```python
from build123d import *

# Parameters (mm, degrees)
BOSS_EXTRUDE1_DEPTH = 7.5
FILLET1_R           = 2.5
SKETCH3_R           = 16.5
BOSS_EXTRUDE2_DEPTH = 5
BOSS_EXTRUDE3_START = -5
BOSS_EXTRUDE3_DEPTH = 5
SKETCH5_R           = 5
BOSS_EXTRUDE4_DEPTH = 10
SKETCH6_R           = 5
CUT_EXTRUDE1_DEPTH  = 10


with BuildPart() as part:
    # Sketch2 → Boss-Extrude1 (new, symmetric)
    with BuildSketch(Plane.XY):
        with BuildLine():
            ThreePointArc((102.783087905, 14.977902914), (19.214406157, 13.934366249), (-64.149557364, 19.872642429))
            ThreePointArc((-64.149557364, 19.872642429), (-86.204808933, 2.808746854), (-69.764850677, -19.715427415))
            ThreePointArc((-69.764850677, -19.715427415), (18.853783166, -25.931146508), (106.966657885, -14.61660998))
            ThreePointArc((106.966657885, -14.61660998), (118.44931566, 2.099570811), (102.783087905, 14.977902914))
        make_face()
    extrude(amount=BOSS_EXTRUDE1_DEPTH, both=True)

    # Fillet1
    fillet1_edges = [part.edges().sort_by_distance(p)[0] for p in [
        (18.853783166, -25.931146508, -7.5),
        (118.44931566, 2.099570811, -7.5),
        (118.44931566, 2.099570811, 7.5),
        (-86.204808933, 2.808746854, -7.5),
        (-86.204808933, 2.808746854, 7.5),
        (19.214406157, 13.934366249, -7.5),
        (19.214406157, 13.934366249, 7.5),
        (18.853783166, -25.931146508, 7.5),
    ]]
    fillet(fillet1_edges, radius=FILLET1_R)

    # Sketch3 → Boss-Extrude2 (add)
    with BuildSketch(Plane.XY.offset(7.5)):
        with Locations((-66.403017571, 0)):
            Circle(SKETCH3_R)
    extrude(amount=BOSS_EXTRUDE2_DEPTH)

    # Sketch4 → Boss-Extrude3 (add)
    with BuildSketch(Plane.XY.offset(12.5).offset(BOSS_EXTRUDE3_START)):
        with BuildLine():
            ThreePointArc((-52.099568751, 8.225652062), (-50.465241438, 4.270514244), (-49.9030415, 0.028100762))
            ThreePointArc((-49.9030415, 0.028100762), (-47.813230422, 1.340878735), (-47.414916211, 3.776457135))
            Line((-47.414916211, 3.776457135), (-48.070610856, 6.223542865))
            ThreePointArc((-48.070610856, 6.223542865), (-49.633350281, 8.133658527), (-52.099568751, 8.225652062))
        make_face()
        with BuildLine():
            ThreePointArc((-54.819051353, -15.511974356), (-53.485336446, -13.435462641), (-54.159948813, -11.061521929))
            ThreePointArc((-54.159948813, -11.061521929), (-57.416473494, -13.838064371), (-61.277519146, -15.683726148))
            ThreePointArc((-61.277519146, -15.683726148), (-59.383205961, -17.265583889), (-56.943747393, -16.891768097))
            Line((-56.943747393, -16.891768097), (-54.819051353, -15.511974356))
        make_face()
        with BuildLine():
            ThreePointArc((-77.576139439, -15.810470249), (-75.18911887, -16.437231094), (-73.139833772, -15.062048582))
            ThreePointArc((-73.139833772, -15.062048582), (-76.786804024, -12.822908364), (-79.735261406, -9.721176591))
            ThreePointArc((-79.735261406, -9.721176591), (-80.654322552, -12.011596414), (-79.544968453, -14.21614395))
            Line((-79.544968453, -14.21614395), (-77.576139439, -15.810470249))
        make_face()
        with BuildLine():
            ThreePointArc((-84.892352865, 5.740566364), (-84.750807928, 3.276695145), (-82.809667718, 1.752663965))
            ThreePointArc((-82.809667718, 1.752663965), (-81.807094609, 5.913071167), (-79.768295833, 9.675708604))
            ThreePointArc((-79.768295833, 9.675708604), (-82.230620043, 9.842009046), (-83.984460073, 8.105707948))
            Line((-83.984460073, 8.105707948), (-84.892352865, 5.740566364))
        make_face()
        with BuildLine():
            ThreePointArc((-66.656933344, 19.358335376), (-68.956474332, 18.462340064), (-69.806068802, 16.145254483))
            ThreePointArc((-69.806068802, 16.145254483), (-65.539474293, 16.477387323), (-61.330969971, 15.701093374))
            ThreePointArc((-61.330969971, 15.701093374), (-61.933708879, 18.094292522), (-64.126995727, 19.225746964))
            Line((-64.126995727, 19.225746964), (-66.656933344, 19.358335376))
        make_face()
    extrude(amount=BOSS_EXTRUDE3_DEPTH)

    # Sketch5 → Boss-Extrude4 (add)
    with BuildSketch(Plane(origin=(0, 0, -7.5), x_dir=(-1, 0, 0), z_dir=(0, 0, -1))):
        with Locations(Location((66.403017571, 0, 0), (0, 0, 180))):
            Circle(SKETCH5_R)
    extrude(amount=BOSS_EXTRUDE4_DEPTH)

    # Sketch6 → Cut-Extrude1 (cut)
    with BuildSketch(Plane.XY.offset(7.5)):
        with Locations((103.596982429, 0)):
            Circle(SKETCH6_R)
    extrude(amount=-CUT_EXTRUDE1_DEPTH, mode=Mode.SUBTRACT)


solid = part.part
```
Here's how the part is built. I have some questions about the finished solid (model axes, mm). A direction names the side the tool comes from. Round coordinates to 2 decimals unless told otherwise and drop trailing zeros. Write each loop counter-clockwise with the first axis right and the second up, starting at its lowest first coordinate (ties: lowest second). Pieces come first, ordered by that corner, then holes. Notation, with made-up numbers: M 22.25,51.25 L 32.25,51.25 A28 cw 32.25,72.25 Z; hole C 86.5,-25 d10. An arc over 180 degrees is marked long. Answer as CSV lines item,"result". Start each with the question number.
1. Thinking about a two-plate mould opening in Y: for faces 1 (the flat face through (-76, 14, 7.5)), 2 (the cylindrical face through (-82.363, -4.188, 9.965)), 3 (the cylindrical face through (-47.833, 1.311, 9.965)), which applies, released by +Y, released by -Y, zero draft, split by the parting line, or undercut?
2. I'm going to push flat-ended pins straight in: pin 1 Ø5 at (x, z) = (37.5, 2) entering from -Y; pin 2 Ø6 at (x, y) = (-1.5, 6.5) entering from +Z; pin 3 Ø12.5 at (x, y) = (7.5, -1.5) entering from -Z. Where does each tip first touch, or does it pass through?
3. On a 3-axis mill with a long thin cutter (end or side, diameter ignored), from which of +Z, -Z, +X, -X, +Y, -Y can I reach the whole of each face in a straight line? I mean faces 4 (the flat face through (-66, 1, 12.5)), 5 (the cylindrical face through (-80.656, -11.976, 9.965)), 6 (the cylindrical face through (-49.602, 8.118, 9.965)), 7 (the cylindrical face through (-67.351, -16.473, 9.965)), 8 (the flat face through (-83.4, 7, 7.5)). Say none if no direction works.
4. Suppose I cut it at A-A on z = -11.5. Write out the boundary of the cut face in (x, y), then the cut area to 3 significant figures.
5. I need wall thicknesses on probe 1 along Z at (x, y) = (29.5, -4.5); probe 2 along Z at (x, y) = (105.5, 0.5); probe 3 along X at (y, z) = (-8, -2.25). Which ranges of each line are inside material? Lowest first, please.
Check result:
1,face 1,"zero draft"
1,face 2,"undercut"
1,face 3,"split by the parting line"
2,pin 1,"stops at y = -25.17"
2,pin 2,"stops at z = 7.5"
2,pin 3,"stops at z = -7.5"
3,face 4,"+Z, +X, -X, +Y, -Y"
3,face 5,"+Z, -X"
3,face 6,"+Z, +Y"
3,face 7,"+Z, -Y"
3,face 8,"none"
4,outline,"C -66.4,0 d10"
4,area,"78.5 mm2"
5,probe 1,"z = -7.5 to 7.5"
5,probe 2,"z = -7.5 to -2.5"
5,probe 3,"x = -84.73 to 116.29"
